from build123d import *
from build123d.topology import SkipClean

# Parameters (mm, degrees)
SKETCH1_R           = 79.871147442
SKETCH1_R_2         = 68.595086453
BOSS_EXTRUDE1_DEPTH = 31
SKETCH2_W           = 233.196890583
SKETCH2_H           = 222.59703192
SKETCH2_W_2         = 56.896718534
SKETCH2_H_2         = 45.723887068
CUT_EXTRUDE1_DEPTH  = 31
BOSS_EXTRUDE2_DEPTH = 5
CUT_EXTRUDE3_DEPTH  = 18
SKETCH6_R           = 9.86264383
CUT_EXTRUDE4_DEPTH  = 128


with BuildPart() as part:
    # Sketch1 → Boss-Extrude1 (new body)
    with BuildSketch(Plane(origin=(0, 0, 0), x_dir=(1, 0, 0), z_dir=(0, 1, 0))):
        with Locations(Location((0, 0, 0), (0, 0, 270))):
            Circle(SKETCH1_R)
        with Locations(Location((0, 0, 0), (0, 0, 270))):
            Circle(SKETCH1_R_2, mode=Mode.SUBTRACT)
    extrude(amount=BOSS_EXTRUDE1_DEPTH)

    # Sketch2 → Cut-Extrude1 (cut)
    with BuildSketch(Plane(origin=(0, 31, 0), x_dir=(1, 0, 0), z_dir=(0, 1, 0))):
        with Locations((-10.138995242, -14.747629444)):
            Rectangle(SKETCH2_W, SKETCH2_H)
        with Locations((0, -68.595086453)):
            Rectangle(SKETCH2_W_2, SKETCH2_H_2, mode=Mode.SUBTRACT)
    extrude(amount=-CUT_EXTRUDE1_DEPTH, mode=Mode.SUBTRACT)

    # Sketch4 → Boss-Extrude2 (add, symmetric)
    with BuildSketch(Plane(origin=(0, 16, 0), x_dir=(1, 0, 0), z_dir=(0, 1, 0))):
        with BuildLine():
            Line((43.392343097, -53.126174774), (39.773823752, -48.69594406))
            ThreePointArc((39.773823752, -48.69594406), (3.024910809, -62.802085461), (-34.909607277, -52.293129027))
            Line((-34.909607277, -52.293129027), (-38.085592821, -57.050622301))
            ThreePointArc((-38.085592821, -57.050622301), (3.30010935, -68.51565634), (43.392343097, -53.126174774))
        make_face()
    extrude(amount=BOSS_EXTRUDE2_DEPTH, both=True)

    # Sketch5 → Cut-Extrude3 (cut)
    with SkipClean():  # the faces are left unmerged after this step: merging them gives an invalid solid
        with BuildSketch(Plane(origin=(0, 21, 0), x_dir=(1, 0, 0), z_dir=(0, 1, 0))):
            with BuildLine():
                ThreePointArc((-20.365734208, -65.502082071), (0, -68.595086453), (20.365734208, -65.502082071))
                Line((20.365734208, -65.502082071), (20.365734208, -59.485198948))
                ThreePointArc((20.365734208, -59.485198948), (0, -62.874891839), (-20.365734208, -59.485198948))
                Line((-20.365734208, -59.485198948), (-20.365734208, -65.502082071))
            make_face()
        extrude(amount=-CUT_EXTRUDE3_DEPTH, mode=Mode.SUBTRACT)

    # Sketch6 → Cut-Extrude4 (cut)
    with SkipClean():  # the faces are left unmerged after this step: merging them gives an invalid solid
        with BuildSketch(Plane.XY):
            with Locations(Location((0, 16, 0), (0, 0, 180))):
                Circle(SKETCH6_R)
        extrude(amount=CUT_EXTRUDE4_DEPTH, mode=Mode.SUBTRACT)


solid = part.part
CAD build for the part. Positions are in the model's coordinates, mm. A direction names the side the tool comes from. Give positions to 0.01 mm unless a question says otherwise; leave off trailing zeros. One line per question, with ' | ' between items. Start each with the question number.
1. Two-plate mould, pull along X, no slides. Class faces 1 (the face through (-20.366, 16, 62)), 2 (the face through (-28.448, 16, 69)), 3 (the face through (0, 31, 73)): pulls with the +X half, pulls with the -X half, needs draft (parallel to the pull), parting line crosses it, or undercut.
2. 3-axis set-ups, long thin cutter, end or side, ignore diameter. For faces 4 (the face through (32, 11, 57)), 5 (the face through (-36.475, 16.07, 54.639)), 6 (the face through (30.686, 16.07, 54.878)), 7 (the face through (32, 21, 57)), 8 (the face through (28.448, 16, 69)): which of +Z, -Z, +X, -X, +Y, -Y reach the whole face in a straight line?
3. Flat gauge pin, fed straight in: pin 1 (5 mm diameter, centred on y = 25.5, z = 53.5, fed in from -X). Where does the tip first touch, or does it go through?
Result sheet:
1) face 1: undercut | face 2: pulls with the -X half | face 3: needs draft
2) face 4: -Z, -Y | face 5: -Z, -X, +Y, -Y | face 6: -Z, +Y, -Y | face 7: -Z, +Y | face 8: +Z, +X, +Y, -Y
3) pin 1: passes through
